Check sheet for the modelled part. Datum: model origin and axes. Units: mm. A direction names the side the tool comes from. Give positions to 0.01 mm unless a question says otherwise; leave off trailing zeros. Loops run counter-clockwise (first coordinate to the right, second up) from the corner with the lowest first, then second, coordinate; pieces in that order, holes last. Notation, with made-up numbers: (40, 45.5) - (73, 45.5) arc R35 ccw to (73, 81.5) - close; hole circle Ø10 at (4.5, 10). An arc over 180 degrees is marked (long way). Answer in a Markdown table with one row per item. Add a question column.
(1) Sectioned sample at A-A on z = 4. Enter the section's corners in (x, y).
(2) Sectioned sample at C-C on y = 2.7. State how many separate pieces and enclosed holes the cut face has, then the cut area to 3 significant figures.
(3) Go/stop test with flat-tipped pins: P1, Ø1, axis at y = -1, z = 31.5, coming from the -X side; P2, Ø3, axis at x = -30, y = 1.5, coming from the +Z side; P3, Ø1.6, axis at x = 15.5, y = 0, coming from the -Z side. Record where each tip stops, or that it passes through.
(4) Thickness scan on L1, parallel to Z at x = -27, y = 2.95; L2, parallel to X at y = 2.4, z = -15; L3, parallel to X at y = 2.45, z = 41. Record the ranges inside material, lowest first.
(5) Draft check along Z on faces 3 (the face through (-39.296, 2, -9)), 4 (the face through (-8, 3.5, -1)), 5 (the face through (15, 1, -10)). Enter one of: released by +Z, released by -Z, zero draft, split by the parting line, or undercut.
(6) Set-up check for faces 1 (the face through (10, 1, 50)), 2 (the face through (-14, 2, -10)): record each of +Z, -Z, +X, -X, +Y, -Y from which the full face is reachable in a straight line by a thin tool's end or side.
(7) Sectioned sample at B-B on x = -12. Enter the section's corners in (y, z), then the cut area to 3 significant figures.
(8) Sectioned sample at D-D on z = 20.5. Enter the section's corners in (x, y).
from build123d import *

# Parameters (mm, degrees)
BOSS_EXTRUDE1_DEPTH = 3.5
BOSS_EXTRUDE3_DEPTH = 2


with BuildPart() as part:
    # Sketch1 → Boss-Extrude1 (new body)
    with BuildSketch(Plane(origin=(0, 0, 0), x_dir=(1, 0, 0), z_dir=(0, 1, 0))):
        Polygon((20, 10), (10, 10), (10, 20), (-50, 20), (-50, 0), (0, 0), (0, -50), (20, -50), align=None)
        Polygon((15.197176758, -43.369163918), (17.5, -45), (15.197176758, -46.630836082), (15.197176758, -45.75), (4.802823242, -45.75), (4.802823242, -46.630836082), (2.5, -45), (4.802823242, -43.369163918), (4.802823242, -44.25), (15.197176758, -44.25), align=None, mode=Mode.SUBTRACT)
        Polygon((7.193827961, -41.21727219), (6.840274571, -40.863718799), (6.48672118, -40.510165409), (9.229988375, -37.766898214), (6.482771236, -34.957244322), (6.840274571, -34.607685506), (7.197777905, -34.25812669), (9.93713979, -37.059746799), (12.742754474, -34.254132115), (13.096307864, -34.607685506), (13.449861255, -34.961238896), (10.636301551, -37.7747986), (13.453811199, -40.656342558), (13.096307864, -41.005901374), (12.73880453, -41.35546019), (9.929150136, -38.481950015), align=None, mode=Mode.SUBTRACT)
        with BuildLine():
            Line((9, -24), (11, -24))
            ThreePointArc((11, -24), (14, -27), (11, -30))
            Line((11, -30), (9, -30))
            ThreePointArc((9, -30), (6, -27), (9, -24))
        make_face(mode=Mode.SUBTRACT)
        Polygon((-43.369163918, 4.802823242), (-45, 2.5), (-46.630836082, 4.802823242), (-45.75, 4.802823242), (-45.75, 15.197176758), (-46.630836082, 15.197176758), (-45, 17.5), (-43.369163918, 15.197176758), (-44.25, 15.197176758), (-44.25, 4.802823242), align=None, mode=Mode.SUBTRACT)
        Polygon((-40.942094571, 12.305355363), (-39.836319425, 10.871595985), (-38.954723638, 12.267051774), (-38.10930457, 11.732948226), (-39.295537885, 9.85528936), (-39.295537885, 7.454795226), (-40.295537885, 7.454795226), (-40.295537885, 9.829586897), (-41.733948351, 11.694644637), align=None, mode=Mode.SUBTRACT)
        with BuildLine():
            ThreePointArc((-30, 11), (-27, 14), (-24, 11))
            Line((-24, 11), (-24, 9))
            ThreePointArc((-24, 9), (-27, 6), (-30, 9))
            Line((-30, 9), (-30, 11))
        make_face(mode=Mode.SUBTRACT)
        with BuildLine():
            Line((8, -10), (12, -10))
            ThreePointArc((12, -10), (14, -12), (12, -14))
            Line((12, -14), (8, -14))
            ThreePointArc((8, -14), (6, -12), (8, -10))
        make_face(mode=Mode.SUBTRACT)
        with BuildLine():
            Line((7, -3), (13, -3))
            ThreePointArc((13, -3), (14, -4), (13, -5))
            Line((13, -5), (7, -5))
            ThreePointArc((7, -5), (6, -4), (7, -3))
        make_face(mode=Mode.SUBTRACT)
        with BuildLine():
            ThreePointArc((-14, 12), (-12, 14), (-10, 12))
            Line((-10, 12), (-10, 8))
            ThreePointArc((-10, 8), (-12, 6), (-14, 8))
            Line((-14, 8), (-14, 12))
        make_face(mode=Mode.SUBTRACT)
        with BuildLine():
            ThreePointArc((-5, 13), (-4, 14), (-3, 13))
            Line((-3, 13), (-3, 7))
            ThreePointArc((-3, 7), (-4, 6), (-5, 7))
            Line((-5, 7), (-5, 13))
        make_face(mode=Mode.SUBTRACT)
    extrude(amount=BOSS_EXTRUDE1_DEPTH)

    # Sketch2 → Boss-Extrude3 (add)
    with BuildSketch(Plane.XZ):
        Polygon((20, 50), (0, 50), (0, 0), (-50, 0), (-50, -20), (10, -20), (10, -10), (20, -10), align=None)
    extrude(amount=BOSS_EXTRUDE3_DEPTH)


solid = part.part
Reply:
| question | item | result |
|---|---|---|
| 1 | outline | (0, -2) - (20, -2) - (20, 3.5) - (14, 3.5) - (14, 0) - (6, 0) - (6, 3.5) - (0, 3.5) - close |
| 2 | separate pieces | 1 |
| 2 | enclosed holes | 10 |
| 2 | area | 2,060 mm^2 |
| 3 | P1 | x = 0 |
| 3 | P2 | z = 0 |
| 3 | P3 | z = -10 |
| 4 | L1 | -20 to -14, -6 to 0 |
| 4 | L2 | -50 to -45.75, -44.25 to 10 |
| 4 | L3 | 0 to 6.98, 7.41 to 12.39, 13.1 to 20 |
| 5 | face 3 | undercut |
| 5 | face 4 | zero draft |
| 5 | face 5 | released by -Z |
| 6 | face 1 | +Z, +X, -X, +Y, -Y |
| 6 | face 2 | +Y |
| 7 | outline | (-2, -20) - (3.5, -20) - (3.5, -14) - (0, -14) - (0, -6) - (3.5, -6) - (3.5, 0) - (-2, 0) - close |
| 7 | area | 82.0 mm^2 |
| 8 | outline | (0, -2) - (20, -2) - (20, 3.5) - (0, 3.5) - close |
